from build123d import *
from build123d.topology import SkipClean

# Parameters (mm, degrees)
BOSS_EXTRUDE1_DEPTH             = 25
BOSS_EXTRUDE2_REACH             = 65.362
BOSS_EXTRUDE2_DIRECTION_2_DEPTH = 30
SKETCH9_R                       = 2.05
CUT_EXTRUDE3_DEPTH              = 35
BOSS_EXTRUDE5_REACH             = 62.904
SKETCH13_R                      = 1.55
CUT_EXTRUDE4_DEPTH              = 87.217897417
SKETCH16_W                      = 50
SKETCH16_H                      = 45
CUT_EXTRUDE5_DEPTH              = 17.5
BOSS_EXTRUDE6_DEPTH             = 17.5
SKETCH20_R                      = 2.05
CUT_EXTRUDE6_DEPTH              = 17.5


with BuildPart() as part:
    # Sketch1 → Boss-Extrude1 (new, symmetric)
    with BuildSketch(Plane.XY):
        with BuildLine():
            Line((-17.5, 22.5), (-17.5, 0))
            Line((-17.5, 0), (17.5, 0))
            Line((17.5, 0), (17.5, 22.5))
            Line((17.5, 22.5), (12.5, 22.5))
            ThreePointArc((12.5, 22.5), (0, 10), (-12.5, 22.5))
            Line((-12.5, 22.5), (-17.5, 22.5))
        make_face()
    boss_extrude1 = extrude(amount=BOSS_EXTRUDE1_DEPTH, both=True)

    # Boss-Extrude2: up to this face of the body (flat: up to its plane)
    boss_extrude2_end = Plane(part.part.faces().sort_by_distance((17.5, 11.25, 0))[0])
    # Sketch5 → Boss-Extrude2 (add, up to the picked face)
    with BuildSketch(Plane(origin=(26.115381057, 0, 15.077722283), x_dir=(0.500000000000001, 0, -0.8660254037844382), z_dir=(0.8660254037844382, 0, 0.500000000000001)), mode=Mode.PRIVATE) as boss_extrude2_sk1:
        with BuildLine():
            Line((-6.7, 22.5), (-3.75, 22.5))
            ThreePointArc((-3.75, 22.5), (8.75, 10), (21.25, 22.5))
            Line((21.25, 22.5), (24.2, 22.5))
            ThreePointArc((24.2, 22.5), (8.75, 7.05), (-6.7, 22.5))
        make_face()
    boss_extrude2_tool1 = split(extrude(boss_extrude2_sk1.sketch, amount=-BOSS_EXTRUDE2_REACH, mode=Mode.PRIVATE), bisect_by=boss_extrude2_end, keep=Keep.BOTH, mode=Mode.PRIVATE)
    boss_extrude2 = boss_extrude2_tool1.solids().sort_by(Axis((23.502881, 22.154527, 19.602705), (-0.8660254037844382, 0, -0.500000000000001)))[0]
    add(boss_extrude2)

    # Sketch5 → Boss-Extrude2 direction 2 (add)
    with BuildSketch(Plane(origin=(26.115381057, 0, 15.077722283), x_dir=(0.500000000000001, 0, -0.8660254037844382), z_dir=(0.8660254037844382, 0, 0.500000000000001))):
        with BuildLine():
            Line((-6.7, 22.5), (-3.75, 22.5))
            ThreePointArc((-3.75, 22.5), (8.75, 10), (21.25, 22.5))
            Line((21.25, 22.5), (24.2, 22.5))
            ThreePointArc((24.2, 22.5), (8.75, 7.05), (-6.7, 22.5))
        make_face()
    boss_extrude2_direction_2 = extrude(amount=BOSS_EXTRUDE2_DIRECTION_2_DEPTH)

    # Sketch9 → Cut-Extrude3 (cut)
    with BuildSketch(Plane.ZY.offset(17.5)):
        with Locations((-18, 5)):
            Circle(SKETCH9_R)
    cut_extrude3 = extrude(amount=-CUT_EXTRUDE3_DEPTH, mode=Mode.SUBTRACT)

    # Boss-Extrude5: up to this face of the body (flat: up to its plane)
    boss_extrude5_end = Plane(part.part.faces().sort_by_distance((17.5, 17.19483523, 0))[0])
    # Sketch12 → Boss-Extrude5 (add, up to the picked face)
    with BuildSketch(Plane(origin=(21.973076211, 0, 12.686161466), x_dir=(0.4999999999999999, 0, -0.8660254037844388), z_dir=(0.8660254037844388, 0, 0.4999999999999999)), mode=Mode.PRIVATE) as boss_extrude5_sk1:
        with BuildLine():
            Line((-3.75, 22.5), (21.25, 22.5))
            ThreePointArc((21.25, 22.5), (8.75, 10), (-3.75, 22.5))
        make_face()
    boss_extrude5_tool1 = split(extrude(boss_extrude5_sk1.sketch, amount=-BOSS_EXTRUDE5_REACH, mode=Mode.PRIVATE), bisect_by=boss_extrude5_end, keep=Keep.BOTH, mode=Mode.PRIVATE)
    boss_extrude5 = boss_extrude5_tool1.solids().sort_by(Axis((26.348076, 17.194835, 5.108439), (-0.8660254037844388, 0, -0.4999999999999999)))[0]
    add(boss_extrude5)

    # Mirror1: Boss-Extrude1, Boss-Extrude2, Boss-Extrude2 direction 2, Cut-Extrude3, Boss-Extrude5 across plane
    with SkipClean():  # the faces are left unmerged after this step: merging them gives an invalid solid
        add(boss_extrude1.mirror(Plane(origin=(17.5, 22.5, 25), x_dir=(0, 0, 1), z_dir=(0, -1, 0))))
        add(boss_extrude2.mirror(Plane(origin=(17.5, 22.5, 25), x_dir=(0, 0, 1), z_dir=(0, -1, 0))))
        add(boss_extrude2_direction_2.mirror(Plane(origin=(17.5, 22.5, 25), x_dir=(0, 0, 1), z_dir=(0, -1, 0))))
        add(cut_extrude3.mirror(Plane(origin=(17.5, 22.5, 25), x_dir=(0, 0, 1), z_dir=(0, -1, 0))), mode=Mode.SUBTRACT)
        add(boss_extrude5.mirror(Plane(origin=(17.5, 22.5, 25), x_dir=(0, 0, 1), z_dir=(0, -1, 0))))

    # Sketch13 → Cut-Extrude4 (cut, through all)
    with SkipClean():  # the faces are left unmerged after this step: merging them gives an invalid solid
        with BuildSketch(Plane(origin=(0, 0, 0), x_dir=(1, 0, 0), z_dir=(0, 1, 0))):
            with Locations(Location((43.480762114, -15, 0), (0, 0, 90))):
                Circle(SKETCH13_R)
        extrude(amount=CUT_EXTRUDE4_DEPTH, mode=Mode.SUBTRACT)

    # Sketch16 → Cut-Extrude5 (cut)
    with SkipClean():  # the faces are left unmerged after this step: merging them gives an invalid solid
        with BuildSketch(Plane(origin=(0, 0, 0), x_dir=(0, 0, -1), z_dir=(1, 0, 0))):
            with Locations((0, 22.5)):
                Rectangle(SKETCH16_W, SKETCH16_H)
        extrude(amount=-CUT_EXTRUDE5_DEPTH, mode=Mode.SUBTRACT)
    add(part.part.scale(1), mode=Mode.REPLACE)  # the faces are merged on a copy

    # Sketch18 → Boss-Extrude6 (add)
    with BuildSketch(Plane.ZY):
        with BuildLine():
            Line((13, 0), (23, 0))
            ThreePointArc((23, 0), (18, -5), (13, 0))
        make_face()
    boss_extrude6 = extrude(amount=-BOSS_EXTRUDE6_DEPTH)

    # Sketch20 → Cut-Extrude6 (cut)
    with BuildSketch(Plane.ZY):
        with Locations((18, 0)):
            Circle(SKETCH20_R)
    cut_extrude6 = extrude(amount=-CUT_EXTRUDE6_DEPTH, mode=Mode.SUBTRACT)

    # Mirror2: Boss-Extrude6, Cut-Extrude6 across plane
    add(boss_extrude6.mirror(Plane.ZX.offset(22.5)))
    add(cut_extrude6.mirror(Plane.ZX.offset(22.5)), mode=Mode.SUBTRACT)


solid = part.part
CAD build for the part. Positions are in the model's coordinates, mm. A direction names the side the tool comes from. Coordinates: 2 decimals unless noted, no trailing zeros. Loops run counter-clockwise (first coordinate to the right, second up) from the corner with the lowest first, then second, coordinate; pieces in that order, holes last. Notation, with made-up numbers: (-25, 3) - (-15, 3) arc R27 cw to (-15, 39) - close; hole circle Ø5 at (7.5, 47). An arc over 180 degrees is marked (long way). Write item = value, one per line. Start each with the question number.
Q1. Cut at B-B, the plane x = 11.5. List the corners of the cut face in (y, z), then the cut area to 3 significant figures.
Q2. Flat gauge pins, fed straight in: pin 1 Ø3.5 at (y, z) = (0, 18) entering from +X; pin 2 Ø3 at (x, z) = (32, 8.5) entering from -Y; pin 3 Ø14 at (x, y) = (8.5, 38.5) entering from +Z; pin 4 Ø1.5 at (x, z) = (12.5, -10.5) entering from -Y. Where does each tip first touch, or does it go through?
Q3. Drill centre lines: L1, parallel to Y at x = 4, z = 18; L2, parallel to X at y = 43, z = 2.5; L3, parallel to Y at x = 29, z = 2. Where is each one in solid material? Low to high.
Q4. Cut at D-D, the plane y = 36.5. List the corners of the cut face in (x, z), then the cut area to 3 significant figures.
Q5. Pull direction Z, two halves, no side cores. Call faces 6 (the flat face through (9, 0, 24)), 7 (the cylindrical face through (44.424, 36.404, 16.23)), 8 (the flat face through (26.436, 22.325, 4.957)), 9 (the cylindrical face through (9, 50, 18)): pulls with the +Z half, pulls with the -Z half, needs draft (parallel to the pull), parting line crosses it, or undercut.
Q6. Cut at C-C, the plane y = 26.5. List the corners of the cut face in (x, z).
Q7. Which spindle directions (+Z, -Z, +X, -X, +Y, -Y) get a long thin tool onto all of the face, cutting with end or side? Do faces 1 (the flat face through (9, 45, -6)), 2 (the flat face through (53.65, 11.13, 27.39)), 3 (the flat face through (9, 0, -6)), 4 (the flat face through (9, 45, 24)), 5 (the cylindrical face through (8.63, 0.09, 15.95)). Say none if no direction does.
Q8. Cut at A-A, the plane y = 5. List the corners of the cut face in (x, z), then the cut area to 3 significant figures.
Computed:
q1.outline = (0, -25) - (17.6, -25) - (17.6, 25) - (0, 25) - (0, 23) arc R5 ccw to (0, 13) - close; (27.4, -25) - (45, -25) - (45, 13) arc R5 ccw to (45, 23) - (45, 25) - (27.4, 25) - close; hole circle Ø4.1 at (0, 18); hole circle Ø4.1 at (5, -18); hole circle Ø4.1 at (40, -18); hole circle Ø4.1 at (45, 18)
q1.area = 1,790 mm²
q2.pin_1 = through
q2.pin_2 = 7.05
q2.pin_3 = 25
q2.pin_4 = 0
q3.L1 = -5 to -2.05, 2.05 to 10.66, 34.34 to 42.95, 47.05 to 50
q3.L2 = 0 to 17.5
q3.L3 = 7.58 to 10.66, 34.34 to 37.42
q4.outline = (0, -25) - (17.5, -25) - (17.5, -7.55) - (59.74, 16.84) - (53.2, 28.16) - (17.5, 7.55) - (17.5, 25) - (0, 25) - close; hole circle Ø3.1 at (43.48, 15)
q4.area = 1,460 mm²
q5.face_6 = needs draft
q5.face_7 = undercut
q5.face_8 = undercut
q5.face_9 = parting line crosses it
q6.outline = (11.84, -25) - (17.5, -25) - (17.5, -17.23) - (63.93, 9.58) - (62.39, 12.24) - (32.27, -5.15) - (20.43, 15.36) - (50.55, 32.76) - (49.01, 35.42) - (17.5, 17.23) - (17.5, 25) - (11.84, 25) - close
q7.face_1 = -Z, +X, -X, +Y
q7.face_2 = +Z, +X, +Y, -Y
q7.face_3 = -Z, +X, -X, -Y
q7.face_4 = +Z, +X, -X, +Y
q7.face_5 = +X, -X
q8.outline = (0, -25) - (17.5, -25) - (17.5, -20.05) - (0, -20.05) - close; (0, -15.95) - (17.5, -15.95) - (17.5, 25) - (0, 25) - close
q8.area = 803 mm²
